```python
from build123d import *

# Parameters (mm, degrees)
BOSS_EXTRUDE1_DEPTH = 130
FILLET1_R           = 50


with BuildPart() as part:
    # Sketch1 → Boss-Extrude1 (new body)
    with BuildSketch(Plane(origin=(0, 0, 0), x_dir=(0, 0, -1), z_dir=(1, 0, 0))):
        Polygon((0, 0), (236, 0), (208, -5), (28, -5), align=None)
    extrude(amount=BOSS_EXTRUDE1_DEPTH)

    # Fillet1
    fillet1_edges = [part.edges().sort_by_distance(p)[0] for p in [
        (65, -5, -208),
        (65, -5, -28),
    ]]
    fillet(fillet1_edges, radius=FILLET1_R)


solid = part.part
```
Input: part model. Units: mm. Frame: model coordinates. Give positions to 0.01 mm unless a question says otherwise; leave off trailing zeros. Order: outer loops, then holes, each group sorted by start corner. A loop starts at its lowest first (then second) coordinate and runs counter-clockwise, first axis right, second up. Notation, with made-up numbers: M 63,6 L 91,6 A32 cw 91,37 Z; hole C 9.5,9.5 d7. An arc over 180 degrees is marked long. One line per question, with ' | ' between items. Start each with the question number.
1. Section query A-A (x = 76.5). Return the cut outline in (y, z), and give its area (3 significant figures).
2. Section query C-C (z = -218). Return the cut outline in (x, y).
3. Material intervals for probe 1 along Y at (x, z) = (48, -28); probe 2 along Y at (x, z) = (21, -214.5), sorted ascending. Write a range as [from, to].
4. Section query B-B (y = -2). Return the cut outline in (x, z).
Here are the results:
1) outline: M -5,-203.57 A50 ccw -4.22,-212.36 L 0,-236 L 0,0 L -4.22,-23.64 A50 ccw -5,-32.43 Z | area: 1,040 mm²
2) outline: M 0,-3.21 L 130,-3.21 L 130,0 L 0,0 Z
3) probe 1: [-4.8, 0] | probe 2: [-3.84, 0]
4) outline: M 0,-224.8 L 130,-224.8 L 130,-11.2 L 0,-11.2 Z
